Geometry: see drawing. Coordinates: mm, zero at the bounding-box minimum. A direction names the side the tool comes from. Coordinates: 2 decimals unless noted, no trailing zeros. Write each loop counter-clockwise with the first axis right and the second up, starting at its lowest first coordinate (ties: lowest second). Pieces come first, ordered by that corner, then holes. Notation, with made-up numbers: M 59.5,18.25 L 72.5,18.25 A31 ccw 72.5,52.25 Z; hole C 72,35.5 d1. An arc over 180 degrees is marked long. Answer as CSV lines item,"result". Start each with the question number.
1. Section D-D on z = 15.5. Return the cut outline in (x, y) (1 decimal), plus the area to 3 significant figures.
2. Contact query for flat-ended pins moving along their axis: pin 1 Ø10 at (x, y) = (10.5, 15) entering from -Z (3 decimals); pin 2 Ø5 at (x, z) = (9.5, 12) entering from -Y; pin 3 Ø5 at (x, y) = (15.5, 4.5) entering from -Z (1 decimal). Output: stop coordinate, or through.
3. Line query: probe 1 along Y at (x, z) = (12.7, 10.75) (1 decimal); probe 2 along X at (y, z) = (4.75, 5.5) (1 decimal). Output: solid intervals per line, ascending. Write a range as [from, to].
4. Mould query, pull axis X, two halves, no side actions, for the marked faces 1, 2 and 3. Classes: pulls with the +X half, pulls with the -X half, needs draft (parallel to the pull), parting line crosses it, or undercut.
5. Reachability of the marked faces 4 and 5 from +Z, -Z, +X, -X, +Y, -Y: full face, straight path, thin tool, end or side. Return the list, or none.
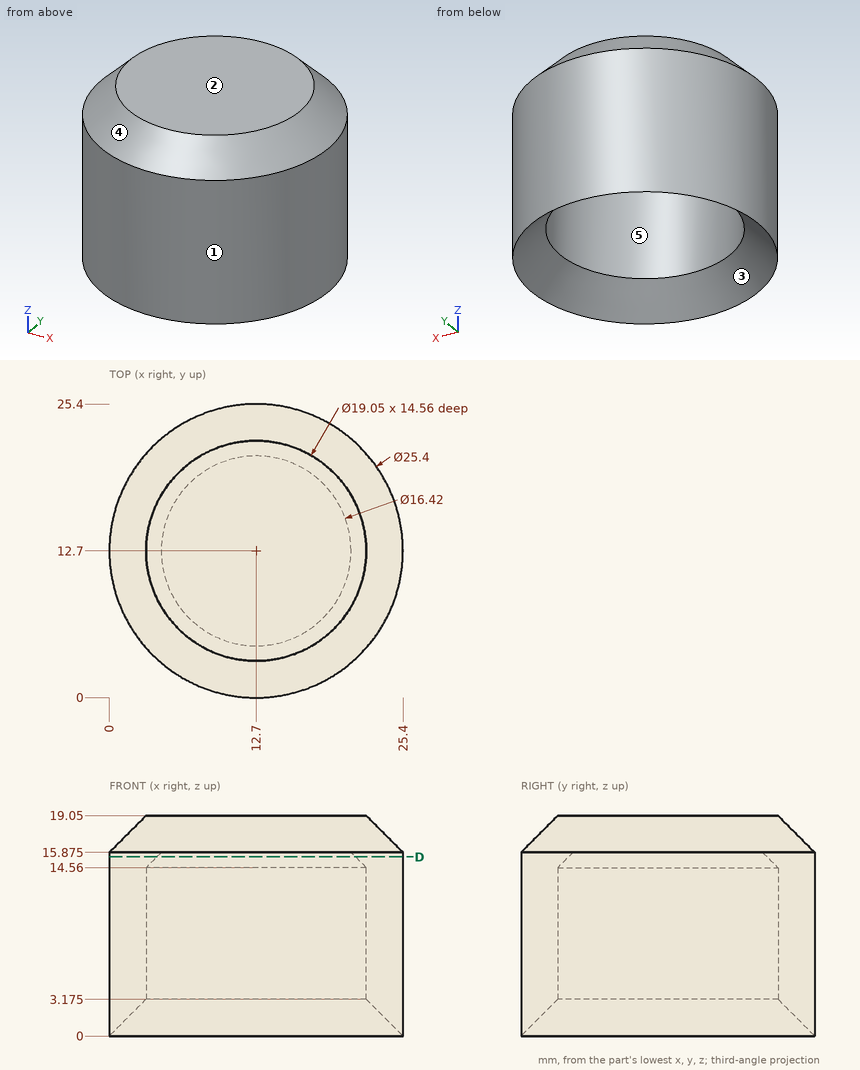
Values:
1,outline,"C 12.7,12.7 d25.4; hole C 12.7,12.7 d17.2"
1,area,"275 mm²"
2,pin 1,"z = 15.875"
2,pin 2,"y = 0.02"
2,pin 3,"z = 1.5"
3,probe 1,"[0, 3.2], [22.2, 25.4]"
3,probe 2,"[2.8, 7.5], [17.9, 22.6]"
4,face 1,"parting line crosses it"
4,face 2,"needs draft"
4,face 3,"undercut"
5,face 4,"+Z"
5,face 5,"-Z"
